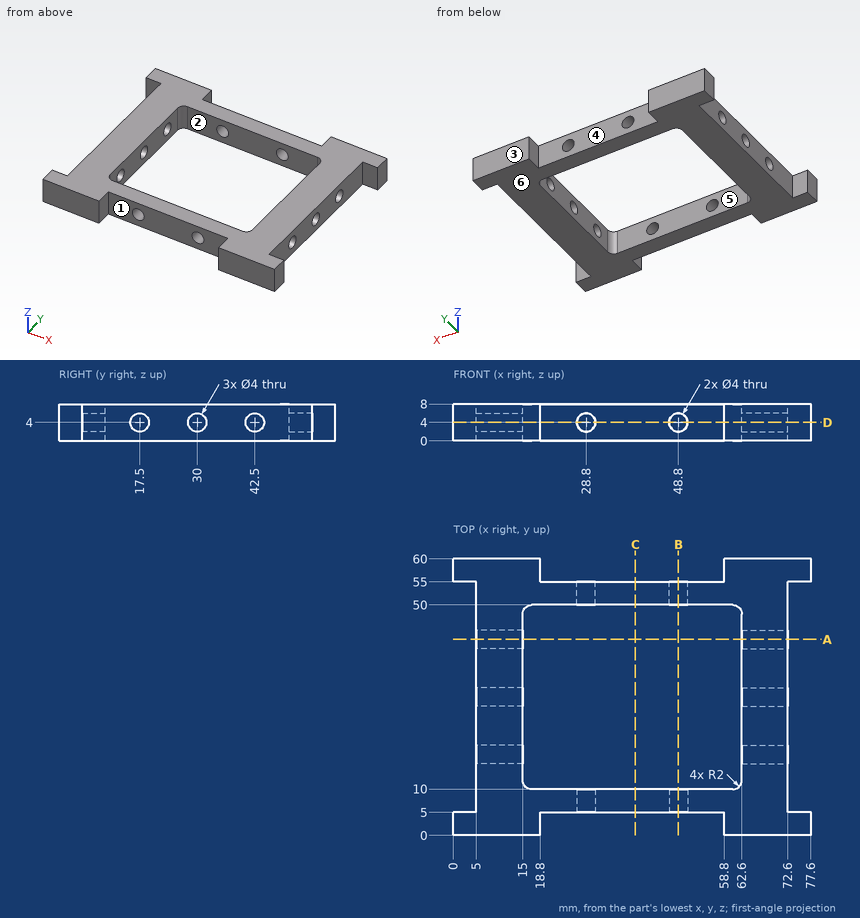
Design review of the part shown in the three views and the two pictorial views. Dimensions are in mm from the part's minimum x, y and z. A direction names the side the tool comes from. Round coordinates to 2 decimals unless told otherwise and drop trailing zeros. Order: outer loops, then holes, each group sorted by start corner. A loop starts at its lowest first (then second) coordinate and runs counter-clockwise, first axis right, second up.
(1) Take a section at A-A, the plane y = 42.5. State the section outline as (x, z) points, plus the area to 3 significant figures.
Working result:
outline: (5, 0) - (15, 0) - (15, 2) - (5, 2) - close; (5, 6) - (15, 6) - (15, 8) - (5, 8) - close; (62.6, 0) - (72.6, 0) - (72.6, 2) - (62.6, 2) - close; (62.6, 6) - (72.6, 6) - (72.6, 8) - (62.6, 8) - close
area: 80.0 mm2
(2) Take a section at D-D, the plane z = 4. Count the separate pieces of the cut face and the enclosed holes in it, plus the area to 3 significant figures.
Working result:
separate pieces: 10
enclosed holes: 0
area: 1,540 mm2
(3) Wall thickness on L1, parallel to Y at x = 66.5, z = 4; L2, parallel to X at y = 51.6, z = 4; L3, parallel to Y at x = 42.5, z = 2.5: over which ranges is each line inside the solid? List them lowest first.
Working result:
L1: y = 0 to 15.5, 19.5 to 28, 32 to 40.5, 44.5 to 60
L2: x = 5 to 26.8, 30.8 to 46.8, 50.8 to 72.6
L3: y = 5 to 10, 50 to 55
(4) Take a section at C-C, the plane x = 39.5. State the section outline as (y, z) points, plus the area to 3 significant figures.
Working result:
outline: (5, 0) - (10, 0) - (10, 8) - (5, 8) - close; (50, 0) - (55, 0) - (55, 8) - (50, 8) - close
area: 80.0 mm2
(5) Take a section at B-B, the plane x = 48.8. State the section outline as (y, z) points.
Working result:
outline: (5, 0) - (10, 0) - (10, 2) - (5, 2) - close; (5, 6) - (10, 6) - (10, 8) - (5, 8) - close; (50, 0) - (55, 0) - (55, 2) - (50, 2) - close; (50, 6) - (55, 6) - (55, 8) - (50, 8) - close
(6) Mouldability with a two-part tool opening along X and no side actions: class the marked faces 1, 2 and 3 as released by +X, released by -X, zero draft, split by the parting line, or undercut.
Working result:
face 1: undercut
face 2: undercut
face 3: zero draft
(7) For P1, Ø2.5, axis at x = 36.5, z = 2.5, coming from the +Y side; P2, Ø1, axis at x = 39.5, y = 12, coming from the +Z side; P3, Ø2.5, axis at y = 21, z = 5.5, coming from the +X side, all flat-tipped, find the tip position at first contact; note any pin that passes through.
Working result:
P1: stops at y = 55
P2: passes through
P3: stops at x = 72.6
(8) Tool access review of the marked faces 4, 5 and 6: name each direction out of +Z, -Z, +X, -X, +Y, -Y from which nothing blocks a thin tool from reaching the whole face with its end or side.
Working result:
face 4: +Z, -Z, +Y
face 5: +Z, -Z
face 6: -Z, +X, -X, +Y, -Y
